from build123d import *

# Parameters (mm, degrees)
F0_W            = 213
F0_H            = 25
F1_DEPTH        = 100
F3_DEPTH        = 20
F4_DEPTH        = 70
F5_R            = 38.333333335
F5_R_2          = 20.5
F6_DEPTH        = 120
F7_R            = 35.5
F7_R_2          = 20.5
F8_DEPTH        = 120
F9_DEPTH        = 213.001
F10_DEPTH       = 200.001
F11_DEPTH       = 10
F13_D           = 14.75
F13_CBORE_D     = 22.25
F13_CBORE_DEPTH = 14
F14_R           = 10


# Not quite as in the source:
# - a fillet or chamfer that OpenCascade refuses, or shapes differently, is made with other operations: its cross-section is extruded or revolved along the edge and cut away or added


with BuildPart() as f1:
    # F0 (on Front) → F1 (new body, symmetric)
    with BuildSketch(Plane.XZ):
        with Locations((0, 12.5)):
            Rectangle(F0_W, F0_H)
    extrude(amount=F1_DEPTH, both=True)

    # F2 (on face) → F3 (cut)
    with BuildSketch(Plane.XY.offset(25)):
        with BuildLine():
            ThreePointArc((-97.5, -21), (-94.5710678119, -28.0710678119), (-87.5, -31))
            Line((-87.5, -31), (-61.5, -31))
            ThreePointArc((-61.5, -31), (-44.5294372515, -38.0294372515), (-37.5, -55))
            Line((-37.5, -55), (-37.5, -81))
            ThreePointArc((-37.5, -81), (-34.5710678119, -88.0710678119), (-27.5, -91))
            Line((-27.5, -91), (29.5, -91))
            ThreePointArc((29.5, -91), (36.5710678119, -88.0710678119), (39.5, -81))
            Line((39.5, -81), (39.5, -51.2013330404))
            ThreePointArc((39.5, -51.2013330404), (37.338740663, -44.9921346366), (31.7891710363, -41.4668738378))
            ThreePointArc((31.7891710363, -41.4668738378), (-19.4358675785, -12.9358675785), (-47.9668738378, 38.2891710363))
            ThreePointArc((-47.9668738378, 38.2891710363), (-51.4921346366, 43.838740663), (-57.7013330404, 46))
            Line((-57.7013330404, 46), (-87.5, 46))
            ThreePointArc((-87.5, 46), (-94.5710678119, 43.0710678119), (-97.5, 36))
            Line((-97.5, 36), (-97.5, -21))
        make_face()
    extrude(amount=-F3_DEPTH, mode=Mode.SUBTRACT)

    # F2 (on face) → F4 (join)
    with BuildSketch(Plane.XY.offset(25)):
        with BuildLine():
            Line((-26.5, 70), (-106.5, 70))
            Line((-106.5, 70), (-106.5, 55))
            Line((-106.5, 55), (-41.5, 55))
            ThreePointArc((-41.5, 55), (-13.0719065478, -6.5719065478), (48.5, -35))
            Line((48.5, -35), (48.5, -100))
            Line((48.5, -100), (63.5, -100))
            Line((63.5, -100), (63.5, -20))
            ThreePointArc((63.5, -20), (-2.46530483, 4.03469517), (-26.5, 70))
        make_face()
    extrude(amount=F4_DEPTH)

    # F5 (on face) → F6 (join)
    with BuildSketch(Plane.XZ.offset(100)):
        with Locations((56, 95)):
            Circle(F5_R)
        with Locations((56, 95)):
            Circle(F5_R_2, mode=Mode.SUBTRACT)
    extrude(amount=-F6_DEPTH)

    # F7 (on face) → F8 (join)
    with BuildSketch(Plane(origin=(-106.5, 0, 0), x_dir=(0, -1, 0), z_dir=(-1, 0, 0))):
        with Locations((-62.5, 95)):
            Circle(F7_R)
        with Locations((-62.5, 95)):
            Circle(F7_R_2, mode=Mode.SUBTRACT)
    extrude(amount=-F8_DEPTH)

    # F7 (on face) → F9 (cut, through all)
    with BuildSketch(Plane(origin=(-106.5, 0, 0), x_dir=(0, -1, 0), z_dir=(-1, 0, 0))):
        with BuildLine():
            ThreePointArc((-42, 95), (-74.0433963806, 111.9410743461), (-70, 75.9212159717))
            Line((-70, 75.9212159717), (-70, 95))
            Line((-70, 95), (-55, 95))
            Line((-55, 95), (-55, 75.9212159717))
            ThreePointArc((-55, 75.9212159717), (-45.5589256539, 83.4566036194), (-42, 95))
        make_face()
        with BuildLine():
            Line((-70, 95), (-70, 75.9212159717))
            ThreePointArc((-70, 75.9212159717), (-62.5, 74.5), (-55, 75.9212159717))
            Line((-55, 75.9212159717), (-55, 95))
            Line((-55, 95), (-70, 95))
        make_face()
    extrude(amount=-F9_DEPTH, mode=Mode.SUBTRACT)

    # F5 (on face) → F10 (cut, through all)
    with BuildSketch(Plane.XZ.offset(100)):
        with BuildLine():
            ThreePointArc((76.5, 95), (44.4566036194, 111.9410743461), (48.5, 75.9212159717))
            Line((48.5, 75.9212159717), (48.5, 95))
            Line((48.5, 95), (63.5, 95))
            Line((63.5, 95), (63.5, 75.9212159717))
            ThreePointArc((63.5, 75.9212159717), (72.9410743461, 83.4566036194), (76.5, 95))
        make_face()
        with BuildLine():
            Line((48.5, 95), (48.5, 75.9212159717))
            ThreePointArc((48.5, 75.9212159717), (56, 74.5), (63.5, 75.9212159717))
            Line((63.5, 75.9212159717), (63.5, 95))
            Line((63.5, 95), (48.5, 95))
        make_face()
    extrude(amount=-F10_DEPTH, mode=Mode.SUBTRACT)

    # F2 (on face) → F11 (join)
    with BuildSketch(Plane.XY.offset(25)):
        with BuildLine():
            Line((-61.5, -40), (-106.5, -40))
            Line((-106.5, -40), (-106.5, -100))
            Line((-106.5, -100), (-46.5, -100))
            Line((-46.5, -100), (-46.5, -55))
            ThreePointArc((-46.5, -55), (-50.8933982822, -44.3933982822), (-61.5, -40))
        make_face()
    extrude(amount=F11_DEPTH)

    # F13 (through all)
    with Locations(Plane.XY.offset(35)):
        with Locations((-76.5, -70)):
            CounterBoreHole(F13_D / 2, F13_CBORE_D / 2, F13_CBORE_DEPTH)

    # F14
    f14_edges = [f1.edges().sort_by_distance(p)[0] for p in [
        (106.5, -100, 12.5),
        (106.5, 100, 12.5),
        (-106.5, 100, 12.5),
        (-106.5, -100, 17.5),
    ]]
    fillet(f14_edges, radius=F14_R)

    # F15: chamfer of 2 on 4 edges, made by hand

    # F15_s1 → F15_t2 (revolve, cut)
    with BuildSketch(Plane.XY.offset(95)):
        Polygon((78.5, -100), (76.5, -98), (76.5, -100), align=None)
    revolve(axis=Axis((56, -100, 95), (0, 1, 0)), mode=Mode.SUBTRACT)

    # F15_s3 → F15_t4 (revolve, cut)
    with BuildSketch(Plane.XY.offset(95)):
        Polygon((-106.5, 40), (-104.5, 42), (-106.5, 42), align=None)
    revolve(axis=Axis((-106.5, 62.5, 95), (1, 0, 0)), mode=Mode.SUBTRACT)

    # F15_s5 → F15_t6 (revolve, cut)
    with BuildSketch(Plane.XY.offset(95)):
        Polygon((11.5, 42), (13.5, 40), (13.5, 42), align=None)
    revolve(axis=Axis((13.5, 62.5, 95), (-1, 0, 0)), mode=Mode.SUBTRACT)

    # F15_s7 → F15_t8 (revolve, cut)
    with BuildSketch(Plane.XY.offset(95)):
        Polygon((76.5, 18), (78.5, 20), (76.5, 20), align=None)
    revolve(axis=Axis((56, 20, 95), (0, -1, 0)), mode=Mode.SUBTRACT)


solid = f1.part
Can you work these out from the model? Positions are in its coordinate system, mm. A direction names the side the tool comes from. Give positions to 0.01 mm unless a question says otherwise; leave off trailing zeros. Loops run counter-clockwise (first coordinate to the right, second up) from the corner with the lowest first, then second, coordinate; pieces in that order, holes last. Notation, with made-up numbers: (19.5, 4) -> (76.5, 4) arc R32 ccw to (76.5, 35) -> close; hole circle Ø10 at (-33, 62). An arc over 180 degrees is marked (long way). Use one line per item in the form item = value.
1) If we section it at D-D (z = 50.5): Please give me the cut outline in (x, y).
Answers:
outline = (-106.5, 55) -> (-41.5, 55) arc R98.12 ccw to (48.5, -35) -> (48.5, -100) -> (63.5, -100) -> (63.5, -20) arc R83.12 cw to (-26.5, 70) -> (-106.5, 70) -> close
2) If we section it at A-A (y = -70): Please give me the cut outline in (x, z) (3 decimals), plus the area to 3 significant figures.
Answers:
outline = (-106.5, 0) -> (-83.875, 0) -> (-83.875, 21) -> (-87.625, 21) -> (-87.625, 35) -> (-106.5, 35) -> close; (-69.125, 0) -> (106.5, 0) -> (106.5, 25) -> (63.5, 25) -> (63.5, 57.408) arc R38.333 ccw (long way) to (48.5, 57.408) -> (48.5, 25) -> (39.5, 25) -> (39.5, 5) -> (-37.5, 5) -> (-37.5, 25) -> (-46.5, 25) -> (-46.5, 35) -> (-65.375, 35) -> (-65.375, 21) -> (-69.125, 21) -> close; hole circle Ø41 at (56, 95)
area = 7,540 mm²
3) Will these pins go through, and if not, where does the flat tip stop? pin 1 (16 mm diameter, centred on x = 1, y = 1, fed in from +Z); pin 2 (6 mm diameter, centred on y = -23, z = 85, fed in from +X); pin 3 (8 mm diameter, centred on y = -86.5, z = 32, fed in from +X).
Answers:
pin_1 = 95
pin_2 = 93.69
pin_3 = 63.5
4) We'd pull the mould along X, two halves only. Please class faces 4 (the face through (-37.5, -68, 15)), 5 (the face through (-103.65, -96.99, 17.74)), 6 (the face through (-84, -40, 30)): released by +X, released by -X, zero draft, split by the parting line, or undercut.
Answers:
face_4 = undercut
face_5 = released by -X
face_6 = zero draft
5) If we section it at B-B (x = -76.5): Please give me the cut outline in (y, z) (3 decimals).
Answers:
outline = (-100, 0) -> (-77.375, 0) -> (-77.375, 21) -> (-81.125, 21) -> (-81.125, 35) -> (-100, 35) -> close; (-62.625, 0) -> (100, 0) -> (100, 25) -> (70, 25) -> (70, 60.301) arc R35.5 ccw (long way) to (55, 60.301) -> (55, 25) -> (46, 25) -> (46, 5) -> (-31, 5) -> (-31, 25) -> (-40, 25) -> (-40, 35) -> (-58.875, 35) -> (-58.875, 21) -> (-62.625, 21) -> close; hole circle Ø41 at (62.5, 95)
6) If we section it at C-C (z = 10): Please give me the cut outline in (x, y) (3 decimals).
Answers:
outline = (-106.5, -90) arc R10 ccw to (-96.5, -100) -> (96.5, -100) arc R10 ccw to (106.5, -90) -> (106.5, 90) arc R10 ccw to (96.5, 100) -> (-96.5, 100) arc R10 ccw to (-106.5, 90) -> close; hole (-97.5, -21) arc R10 ccw to (-87.5, -31) -> (-61.5, -31) arc R24 cw to (-37.5, -55) -> (-37.5, -81) arc R10 ccw to (-27.5, -91) -> (29.5, -91) arc R10 ccw to (39.5, -81) -> (39.5, -51.201) arc R10 ccw to (31.789, -41.467) arc R107.123 cw to (-47.967, 38.289) arc R10 ccw to (-57.701, 46) -> (-87.5, 46) arc R10 ccw to (-97.5, 36) -> close; hole circle Ø14.75 at (-76.5, -70)
7) I need wall thicknesses on line 1 along Y through (x, z) = (-76.5, 27.75) (3 decimals); line 2 along Y through (x, z) = (-76.5, 11) (3 decimals); line 3 along Z through (x, y) = (-44, 62). Which ranges of each line are inside material? Lowest first, please.
Answers:
line_1 = -100 to -81.125, -58.875 to -40, 55 to 70
line_2 = -100 to -77.375, -62.625 to -31, 46 to 100
line_3 = 0 to 74.51, 115.49 to 130.5
8) For faces 1 (the face through (-9, 0, 95)), 2 (the face through (-66, 70, 42)), 3 (the face through (-34.65, -87.99, 15.14)), which set-ups out of +Z, -Z, +X, -X, +Y, -Y let a thin tool reach every point of the face, with its end or its side?
Answers:
face_1 = +Z, -X, -Y
face_2 = +X, -X, +Y
face_3 = +Z
